Source: three-view drawing plus pictorial views. Frame: mm from the lowest corner of the part. A direction names the side the tool comes from. Give positions to 0.01 mm unless a question says otherwise; leave off trailing zeros. Write each loop counter-clockwise with the first axis right and the second up, starting at its lowest first coordinate (ties: lowest second). Pieces come first, ordered by that corner, then holes. Notation, with made-up numbers: (82, -10.5) -> (134, -10.5) arc R5 ccw to (134, -2.5) -> close; hole circle Ø1 at (10, -25.5). An arc over 180 degrees is marked (long way). Answer in a Markdown table with one row per item. Add a question column.
Item 1: First-contact query: P1, Ø7.5, axis at x = 3, z = 40, coming from the +Y side; P2, Ø7.5, axis at x = 69.5, z = 31.5, coming from the +Y side; P3, Ø9, axis at y = 11, z = 26.5, coming from the +X side; P4, Ø3, axis at y = 24, z = 65.5, coming from the -X side. Flat tips, straight axial feed; report the tip coordinate or a pass-through.
Item 2: Material intervals for probe 1 along X at (y, z) = (1.35, 37); probe 2 along Z at (x, y) = (69.5, 1.35); probe 3 along X at (y, z) = (19.5, 22), sorted ascending. Write a range as from..to.
Item 3: Section query D-D on y = 15.5. Output: boundary loops of the cut face in (x, z), plus the area to 3 significant figures.
Item 4: Section query B-B on x = 4.5. Output: boundary loops of the cut face in (y, z).
Item 5: Section query A-A on z = 37. Output: boundary loops of the cut face in (x, y), plus the area to 3 significant figures.
Item 6: Section query C-C on z = 22. Output: boundary loops of the cut face in (x, y).
Item 7: Draft query along Z for the marked faces 1, 2 and 3. Return one class per face: +Z half, -Z half, draft (parallel to the pull), parting line (faces both ways), or undercut.
Item 8: Access query for the marked faces 4 and 5. Directions: +Z, -Z, +X, -X, +Y, -Y. A direction counts if a zero-diameter tool reaches every point of the face in a straight line with its end or side. Return the directions, or none.
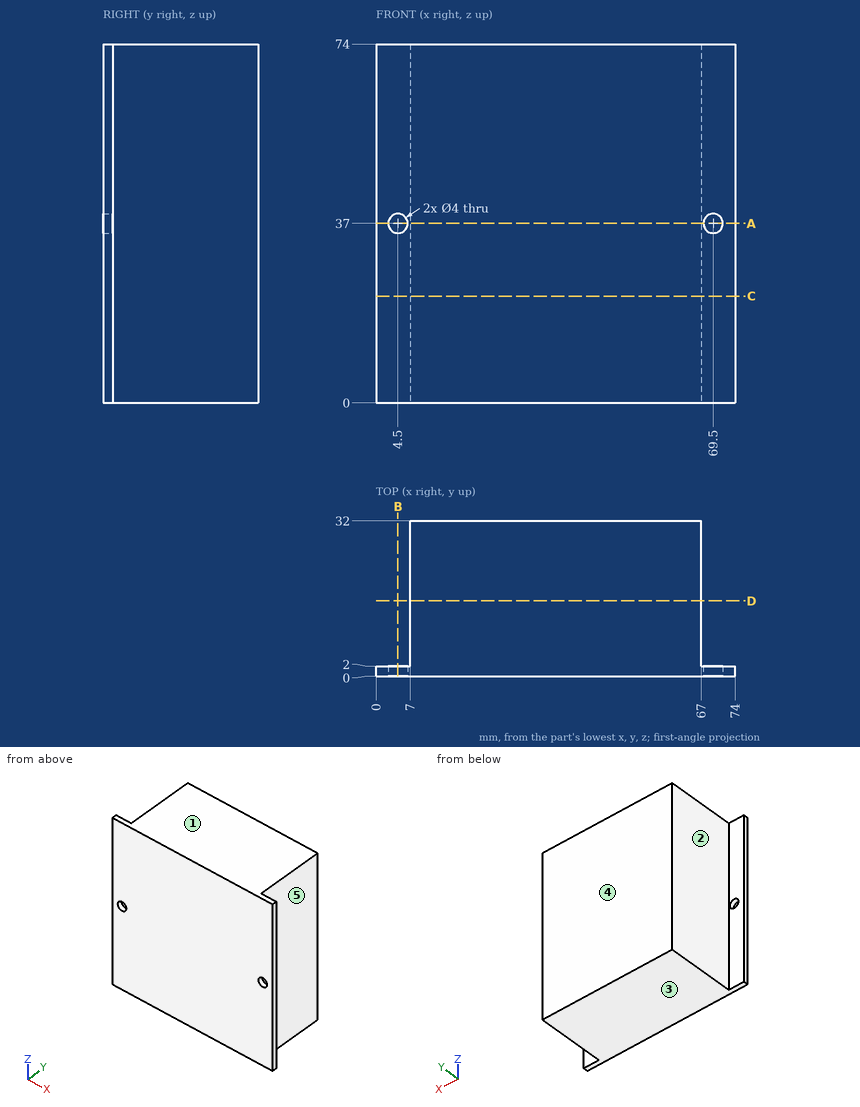
Findings below:
| question | item | result |
|---|---|---|
| 1 | P1 | stops at y = 2 |
| 1 | P2 | stops at y = 32 |
| 1 | P3 | stops at x = 67 |
| 1 | P4 | stops at x = 7 |
| 2 | probe 1 | x = 0..2.5, 6.5..67.5, 71.5..74 |
| 2 | probe 2 | z = 0..35, 39..74 |
| 2 | probe 3 | x = 7..67 |
| 3 | outline | (7, 0) -> (67, 0) -> (67, 74) -> (7, 74) -> close |
| 3 | area | 4,440 mm^2 |
| 4 | outline | (0, 0) -> (2, 0) -> (2, 35) -> (0, 35) -> close; (0, 39) -> (2, 39) -> (2, 74) -> (0, 74) -> close |
| 5 | outline | (0, 0) -> (2.5, 0) -> (2.5, 2) -> (0, 2) -> close; (6.5, 0) -> (67.5, 0) -> (67.5, 2) -> (67, 2) -> (67, 32) -> (7, 32) -> (7, 2) -> (6.5, 2) -> close; (71.5, 0) -> (74, 0) -> (74, 2) -> (71.5, 2) -> close |
| 5 | area | 1,930 mm^2 |
| 6 | outline | (0, 0) -> (74, 0) -> (74, 2) -> (67, 2) -> (67, 32) -> (7, 32) -> (7, 2) -> (0, 2) -> close |
| 7 | face 1 | +Z half |
| 7 | face 2 | draft |
| 7 | face 3 | -Z half |
| 8 | face 4 | +Z, -Z, +X, -X, +Y |
| 8 | face 5 | +Z, -Z, +X, +Y |
